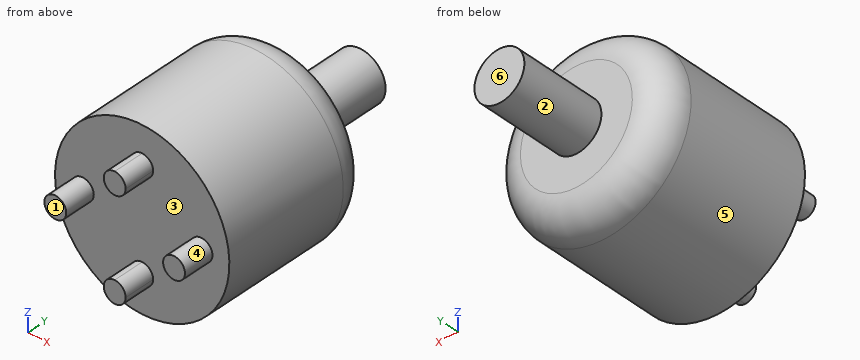
```python
from build123d import *

# Parameters (mm, degrees)
SKETCH1_R           = 13.95
BOSS_EXTRUDE1_DEPTH = 25.7
FILLET1_R           = 5
SKETCH2_R           = 4
BOSS_EXTRUDE2_DEPTH = 14
BOSS_EXTRUDE3_DEPTH = 5


with BuildPart() as part:
    # Sketch1 → Boss-Extrude1 (new body)
    with BuildSketch(Plane(origin=(0, 0, 0), x_dir=(1, 0, 0), z_dir=(0, 1, 0))):
        with Locations(Location((0, 0, 0), (0, 0, 90))):
            Circle(SKETCH1_R)
    extrude(amount=BOSS_EXTRUDE1_DEPTH)

    # Fillet1
    fillet1_edges = [part.edges().sort_by_distance(p)[0] for p in [
        (0, 25.7, 13.95),
    ]]
    fillet(fillet1_edges, radius=FILLET1_R)

    # Sketch2 → Boss-Extrude2 (add)
    with BuildSketch(Plane(origin=(0, 25.7, 0), x_dir=(1, 0, 0), z_dir=(0, 1, 0))):
        with Locations(Location((0, 0, 0), (0, 0, 270))):
            Circle(SKETCH2_R)
    extrude(amount=BOSS_EXTRUDE2_DEPTH)

    # Sketch3 → Boss-Extrude3 (add)
    with BuildSketch(Plane.XZ):
        with BuildLine():
            ThreePointArc((0, 9.75), (-1.75, 8), (0, 6.25))
            Line((0, 6.25), (0, 9.75))
        make_face()
        with BuildLine():
            Line((0, 9.75), (0, 6.25))
            ThreePointArc((0, 6.25), (1.237436867, 6.762563133), (1.75, 8))
            ThreePointArc((1.75, 8), (1.237436867, 9.237436867), (0, 9.75))
        make_face()
        with BuildLine():
            ThreePointArc((-11.25, 0), (-9.5, -1.75), (-7.75, 0))
            Line((-7.75, 0), (-11.25, 0))
        make_face()
        with BuildLine():
            Line((-11.25, 0), (-7.75, 0))
            ThreePointArc((-7.75, 0), (-9.5, 1.75), (-11.25, 0))
        make_face()
        with BuildLine():
            ThreePointArc((1.75, -8), (1.237436867, -6.762563133), (0, -6.25))
            Line((0, -6.25), (0, -9.75))
            ThreePointArc((0, -9.75), (1.237436867, -9.237436867), (1.75, -8))
        make_face()
        with BuildLine():
            Line((0, -9.75), (0, -6.25))
            ThreePointArc((0, -6.25), (-1.75, -8), (0, -9.75))
        make_face()
        with BuildLine():
            ThreePointArc((7.75, 0), (9.5, -1.75), (11.25, 0))
            Line((11.25, 0), (7.75, 0))
        make_face()
        with BuildLine():
            Line((7.75, 0), (11.25, 0))
            ThreePointArc((11.25, 0), (9.5, 1.75), (7.75, 0))
        make_face()
    extrude(amount=BOSS_EXTRUDE3_DEPTH)


solid = part.part
```
Source: CAD feature listing. Evaluate the final solid. Frame: model axes, mm. Face numbers are marked on the shaded views. A direction names the side the tool comes from. Give positions to 0.01 mm unless a question says otherwise; leave off trailing zeros. Order: outer loops, then holes, each group sorted by start corner. A loop starts at its lowest first (then second) coordinate and runs counter-clockwise, first axis right, second up.
(1) Pull-direction query (X, two-part tool) for the marked faces 4, 5 and 6; classes: +X half, -X half, draft (parallel to the pull), parting line (faces both ways), or undercut.
(2) Material intervals for line 1 along Y through (x, z) = (2.75, -7.25); line 2 along Y through (x, z) = (0, -3.5); line 3 along Z through (x, y) = (1.5, 25), sorted ascending.
(3) Contact query for flat-ended pins moving along their axis: P1, Ø10, axis at x = 6.5, y = 5.5, coming from the +Z side; P2, Ø3, axis at y = 11, z = -4.5, coming from the +X side; P3, Ø8, axis at x = -11, z = -7.5, coming from the -Y side. Output: stop coordinate, or through.
(4) Section query A-A (z = 0). Return the cut outline in (x, y).
(5) Access query for the marked faces 1, 2 and 3. Directions: +Z, -Z, +X, -X, +Y, -Y. A direction counts if a zero-diameter tool reaches every point of the face in a straight line with its end or side. Return the directions, or none.
(6) Section query B-B (y = 29.5). Return the cut outline in (x, z).
Outcome:
1. face 4: undercut
1. face 5: parting line
1. face 6: draft
2. line 1: y = 0 to 25.7
2. line 2: y = 0 to 39.7
2. line 3: z = -11.4 to 11.4
3. P1: stops at z = 13.87
3. P2: stops at x = 13.62
3. P3: stops at y = 0
4. outline: (-13.95, 0) - (-11.25, 0) - (-11.25, -5) - (-7.75, -5) - (-7.75, 0) - (7.75, 0) - (7.75, -5) - (11.25, -5) - (11.25, 0) - (13.95, 0) - (13.95, 20.7) arc R5 ccw to (8.95, 25.7) - (4, 25.7) - (4, 39.7) - (-4, 39.7) - (-4, 25.7) - (-8.95, 25.7) arc R5 ccw to (-13.95, 20.7) - close
5. face 1: +Z, -Z, +X, -X, -Y
5. face 2: +Y
5. face 3: -Y
6. outline: circle Ø8 at (0, 0)
